Read the model definition and answer for the solid it produces. Units are mm, in the model's axes. A direction names the side the tool comes from. Coordinates: 2 decimals unless noted, no trailing zeros. Write each loop counter-clockwise with the first axis right and the second up, starting at its lowest first coordinate (ties: lowest second). Pieces come first, ordered by that corner, then holes.
(1) Determine the mould class of faces 4 (the flat face through (14, 1, 0)), 5 (the cylindrical face through (1.3, 3.5, 8)), 6 (the flat face through (-20, 0, 17)) for opening direction X: pulls with the +X half, pulls with the -X half, needs draft (parallel to the pull), parting line crosses it, or undercut.
(2) The part is cut by section C-C, the plane y = -1.25. Determine the outline of the cut face in (x, z).
(3) Which of the six approach directions +Z, -Z, +X, -X, +Y, -Y give full straight-line access (tool end or side, diameter ignored) to faces 1 (the flat face through (0, -4, 6)), 2 (the cylindrical face through (1.34, -1.04, 6)), 3 (the flat face through (0, 2, 6))?
(4) The part is cut by section B-B, the plane y = 3.25. Determine the outline of the cut face in (x, z), and give its area (3 significant figures).
(5) The part is cut by section A-A, the plane x = 2.5. Determine the outline of the cut face in (y, z).
(6) Straight lines are drawn through the part: line 1 along Z through (x, y) = (1.5, 0.75); line 2 along X through (y, z) = (3, 4.5); line 3 along Z through (x, y) = (-5.5, 2.5). For each, find the intervals that lie inside material, in ascending order.
(7) Given pin 1 (2.5 mm diameter, centred on x = 4, z = 4.5, fed in from +Y); pin 2 (2 mm diameter, centred on x = -14.5, y = -1.5, fed in from -Z); pin 3 (1.5 mm diameter, centred on x = -0.5, y = -2.5, fed in from -Z), each flat-ended and moving along its own axis, determine where each tip first touches the part or whether it passes through.
```python
from build123d import *

# Parameters (mm, degrees)
SKETCH1_W           = 40
SKETCH1_H           = 9.108063915
BOSS_EXTRUDE1_DEPTH = 35
CAVITY1_START       = -4.108063915
CAVITY1_DEPTH       = 9.108063915
CAVITY1_START_2     = 2
CAVITY1_2_DEPTH     = 3
CAVITY1_3_DEPTH     = 0.108063915


# Read off the part's stored shape, not the designer's step: Cavity1
with BuildPart() as part:
    # Sketch1 → Boss-Extrude1 (new body)
    with BuildSketch(Plane.XY):
        with Locations((0, 0.445968042)):
            Rectangle(SKETCH1_W, SKETCH1_H)
    extrude(amount=BOSS_EXTRUDE1_DEPTH)

    # Cavity1 outline → Cavity1 (cut)
    with BuildSketch(Plane(origin=(0, 0, 0), x_dir=(1, 0, 0), z_dir=(0, 1, 0)).offset(CAVITY1_START)):
        with BuildLine():
            ThreePointArc((-4.532210811, 0), (1.467789189, -6), (7.467789189, 0))
            Line((7.467789189, 0), (-4.532210811, 0))
        make_face()
    extrude(amount=CAVITY1_DEPTH, mode=Mode.SUBTRACT)

    # Cavity1 2 outline → Cavity1 2 (cut)
    with BuildSketch(Plane(origin=(0, 0, 0), x_dir=(1, 0, 0), z_dir=(0, 1, 0)).offset(CAVITY1_START_2)):
        with BuildLine():
            ThreePointArc((-6.532210811, 0), (1.467789189, -8), (9.467789189, 0))
            Line((9.467789189, 0), (7.467789189, 0))
            ThreePointArc((7.467789189, 0), (1.467789189, -6), (-4.532210811, 0))
            Line((-4.532210811, 0), (-6.532210811, 0))
        make_face()
    extrude(amount=CAVITY1_2_DEPTH, mode=Mode.SUBTRACT)

    # Cavity1 3 outline → Cavity1 3 (cut)
    with BuildSketch(Plane(origin=(0, 0, 0), x_dir=(1, 0, 0), z_dir=(0, 1, 0)).offset(CAVITY1_START)):
        with BuildLine():
            ThreePointArc((-6.532210811, 0), (1.467789189, -8), (9.467789189, 0))
            Line((9.467789189, 0), (7.467789189, 0))
            ThreePointArc((7.467789189, 0), (1.467789189, -6), (-4.532210811, 0))
            Line((-4.532210811, 0), (-6.532210811, 0))
        make_face()
    extrude(amount=CAVITY1_3_DEPTH, mode=Mode.SUBTRACT)


solid = part.part
```
Computed:
1. face 4: needs draft
1. face 5: undercut
1. face 6: pulls with the -X half
2. outline: (-20, 0) - (-4.53, 0) arc R6 cw to (7.47, 0) - (20, 0) - (20, 35) - (-20, 35) - close
3. face 1: -Z, -Y
3. face 2: -Z, +Y, -Y
3. face 3: -Z, +Y
4. outline: (-20, 0) - (-6.53, 0) arc R8 cw to (9.47, 0) - (20, 0) - (20, 35) - (-20, 35) - close
4. area: 1,300 mm2
5. outline: (-4.11, 7.93) - (-4, 7.93) - (-4, 5.91) - (2, 5.91) - (2, 7.93) - (5, 7.93) - (5, 35) - (-4.11, 35) - close
6. line 1: z = 6 to 35
6. line 2: x = -20 to -5.15, 8.08 to 20
6. line 3: z = 3.93 to 35
7. pin 1: stops at y = 2
7. pin 2: stops at z = 0
7. pin 3: stops at z = 5.35
